CAD build for the part. Positions are in the model's coordinates, mm. A direction names the side the tool comes from. Round coordinates to 2 decimals unless told otherwise and drop trailing zeros. Loops run counter-clockwise (first coordinate to the right, second up) from the corner with the lowest first, then second, coordinate; pieces in that order, holes last. Notation, with made-up numbers: (33.25, 8) - (78.25, 8) arc R29 ccw to (78.25, 33) - close; hole circle Ø9 at (30.5, -15). An arc over 180 degrees is marked (long way). One line per question, with ' | ' between items.
```python
from build123d import *

# Parameters (mm, degrees)
BOSS_EXTRUDE1_DEPTH = 1.2
SKETCH2_R           = 5.35
BOSS_EXTRUDE2_DEPTH = 1.9
SKETCH3_R           = 3.4
BOSS_EXTRUDE3_DEPTH = 6.1
FILLET2_R           = 0.8
SKETCH4_R           = 3
BOSS_EXTRUDE4_DEPTH = 8.9
SKETCH5_R           = 8.25
BOSS_EXTRUDE5_DEPTH = 5.9
FILLET1_R           = 0.8
SKETCH6_W           = 12.99598454
SKETCH6_H           = 2
BOSS_EXTRUDE6_DEPTH = 5.9
FILLET3_R           = 0.6
CHAMFER1_SIZE       = 2
BOSS_EXTRUDE7_DEPTH = 4.4
FILLET4_R           = 0.2


with BuildPart() as part:
    # Sketch1 → Boss-Extrude1 (new body)
    with BuildSketch(Plane.XY):
        with BuildLine():
            Line((7.5, -4), (7.5, -16.5))
            Line((7.5, -16.5), (-7.5, -16.5))
            Line((-7.5, -16.5), (-7.5, -4))
            ThreePointArc((-7.5, -4), (0, 8.5), (7.5, -4))
        make_face()
    extrude(amount=BOSS_EXTRUDE1_DEPTH)

    # Sketch2 → Boss-Extrude2 (add)
    with BuildSketch(Plane.XY.offset(1.2)):
        with Locations(Location((0, 0, 0), (0, 0, 180))):
            Circle(SKETCH2_R)
    extrude(amount=BOSS_EXTRUDE2_DEPTH)

    # Sketch3 → Boss-Extrude3 (add)
    with BuildSketch(Plane.XY.offset(3.1)):
        Circle(SKETCH3_R)
    extrude(amount=BOSS_EXTRUDE3_DEPTH)

    # Fillet2
    fillet2_edges = [part.edges().sort_by_distance(p)[0] for p in [
        (-3.4, 0, 9.2),
    ]]
    fillet(fillet2_edges, radius=FILLET2_R)

    # Sketch4 → Boss-Extrude4 (add)
    with BuildSketch(Plane.XY.offset(9.2)):
        Circle(SKETCH4_R)
    extrude(amount=BOSS_EXTRUDE4_DEPTH)

    # Sketch5 → Boss-Extrude5 (add)
    with BuildSketch(Plane(origin=(0, 0, 0), x_dir=(-1, 0, 0), z_dir=(0, 0, -1))):
        with Locations(Location((0, 0, 0), (0, 0, 180))):
            Circle(SKETCH5_R)
    extrude(amount=BOSS_EXTRUDE5_DEPTH)

    # Fillet1
    fillet1_edges = [part.edges().sort_by_distance(p)[0] for p in [
        (-8.25, 0, -5.9),
    ]]
    fillet(fillet1_edges, radius=FILLET1_R)

    # Sketch6 → Boss-Extrude6 (add)
    with BuildSketch(Plane(origin=(0, 0, 0), x_dir=(-1, 0, 0), z_dir=(0, 0, -1))):
        with Locations((0, -10)):
            Rectangle(SKETCH6_W, SKETCH6_H)
    extrude(amount=BOSS_EXTRUDE6_DEPTH)

    # Fillet3
    # the kernel refuses this fillet: 0.6 mm, written as the material it takes off along each edge
    with BuildSketch(Plane(origin=(0, 0, 9.2), x_dir=(1, 0, 0), z_dir=(0, -1, 0))) as fillet3_piece_1:
        with BuildLine():
            CenterArc((2.4, 0.565685425), FILLET3_R, 289.471220634, 70.528779366)
            Line((3, 0.565685425), (3, 0))
            Line((3, 0), (2.6, 0))
        make_face()
    revolve(axis=Axis((0, 0, 9.2), (0, 0, 1)), mode=Mode.SUBTRACT)
    with BuildSketch(Plane(origin=(0, 0, 18.1), x_dir=(1, 0, 0), z_dir=(0, -1, 0))) as fillet3_piece_2:
        with BuildLine():
            CenterArc((3 - FILLET3_R, -FILLET3_R), FILLET3_R, 0, 90)
            Line((3 - FILLET3_R, 0), (3, 0))
            Line((3, 0), (3, -FILLET3_R))
        make_face()
    revolve(axis=Axis((0, 0, 18.1), (0, 0, 1)), mode=Mode.SUBTRACT)

    # Chamfer1
    chamfer1_edges = [part.edges().sort_by_distance(p)[0] for p in [
        (7.5, -16.5, 0.6),
        (-7.5, -16.5, 0.6),
    ]]
    chamfer(chamfer1_edges, length=CHAMFER1_SIZE)

    # Sketch8 → Boss-Extrude7 (add)
    with BuildSketch(Plane.XY.offset(1.2)):
        with BuildLine():
            Line((-8.40758586, 1.25), (-7.293661632, 1.25))
            ThreePointArc((-7.293661632, 1.25), (-7.4, 0), (-7.293661632, -1.25))
            Line((-7.293661632, -1.25), (-8.40758586, -1.25))
            ThreePointArc((-8.40758586, -1.25), (-8.5, 0), (-8.40758586, 1.25))
        make_face()
    extrude(amount=BOSS_EXTRUDE7_DEPTH)

    # Fillet4
    fillet4_edges = [part.edges().sort_by_distance(p)[0] for p in [
        (-8.40758586, 1.25, 3.4),
        (-8.40758586, -1.25, 3.4),
        (-7.293661632, -1.25, 3.4),
        (-7.293661632, 1.25, 3.4),
    ]]
    fillet(fillet4_edges, radius=FILLET4_R)


solid = part.part
```
(1) Cut at A-A, the plane y = 0. Write the cut outline in (x, z).
Results found:
outline: (-8.5, 0) - (-8.25, 0) - (-8.25, -5.1) arc R0.8 ccw to (-7.45, -5.9) - (7.45, -5.9) arc R0.8 ccw to (8.25, -5.1) - (8.25, 0) - (8.5, 0) - (8.5, 1.2) - (5.35, 1.2) - (5.35, 3.1) - (3.4, 3.1) - (3.4, 8.4) arc R0.8 ccw to (2.6, 9.2) arc R0.6 ccw to (3, 9.77) - (3, 17.5) arc R0.6 ccw to (2.4, 18.1) - (-2.4, 18.1) arc R0.6 ccw to (-3, 17.5) - (-3, 9.77) arc R0.6 ccw to (-2.6, 9.2) arc R0.8 ccw to (-3.4, 8.4) - (-3.4, 3.1) - (-5.35, 3.1) - (-5.35, 1.2) - (-7.4, 1.2) - (-7.4, 5.6) - (-8.5, 5.6) - close
(2) Cut at C-C, the plane y = -10. Write the cut outline in (x, z), then the cut area to 3 significant figures.
Results found:
outline: (-7.5, 0) - (-6.5, 0) - (-6.5, -5.9) - (6.5, -5.9) - (6.5, 0) - (7.5, 0) - (7.5, 1.2) - (-7.5, 1.2) - close | area: 94.7 mm²
(3) Probe L1, parallel to Z at x = -5.5, y = -14; L2, parallel to Z at x = 4.5, y = -0.5; L3, parallel to Y at x = -4.75, z = -0.25. List the from-to ranges inside material, lowest first.
Results found:
L1: z = 0 to 1.2 | L2: z = -5.9 to 3.1 | L3: y = -11 to -9, -6.75 to 6.75
(4) Tool access for faces 1 (the face through (-0.74, -3.32, 5.71)), 2 (the face through (-6.498, -10, -3)), 3 (the face through (7.5, -9, 1)), 4 (the face through (6.498, -10, -3)), 5 (the face through (7.87, -2.48, -2.51)): list every direction of +Z, -Z, +X, -X, +Y, -Y with a clear straight run to the whole face (end or side of a thin tool).
Results found:
face 1: +Z | face 2: -Z, -X, -Y | face 3: +Z, -Z, +X, -Y | face 4: -Z, +X, -Y | face 5: -Z
(5) Drop flat-ended pins along their axis: P1, Ø0.6, axis at x = -8, y = 0, coming from the +Z side; P2, Ø1.6, axis at y = -9.5, z = -3.5, coming from the -X side; P3, Ø0.6, axis at x = -8, z = 4, coming from the -Y side. Give the stop position or say it passes through.
Results found:
P1: stops at z = 5.6 | P2: stops at x = -6.5 | P3: stops at y = -1.25
(6) Two-plate mould, pull along X, no slides. Class faces 6 (the face through (-7.5, -9, 1)), 7 (the face through (0, -11, -3)), 8 (the face through (-7.4, 0, 3.4)), 9 (the face through (-3, 0, 14)): released by +X, released by -X, zero draft, split by the parting line, or undercut.
Results found:
face 6: released by -X | face 7: zero draft | face 8: undercut | face 9: split by the parting line
